```python
from build123d import *

# Parameters (mm, degrees)
BOSS_EXTRUDE1_DEPTH = 2
FILLET1_R           = 1
FILLET2_R           = 5
FILLET3_R           = 9


with BuildPart() as part:
    # Sketch1 → Boss-Extrude1 (new body)
    with BuildSketch(Plane(origin=(0, 0, 0), x_dir=(1, 0, 0), z_dir=(0, 1, 0))):
        Polygon((3, 0), (5, 0), (10, 11.071428571), (15, 0), (17, 0), (17, -5), (20, -5), (20, 0), (20, 2), (13, 17.5), (20, 33), (20, 35), (20, 40), (17, 40), (17, 35), (15, 35), (10, 23.928571429), (5, 35), (3, 35), (3, 40), (0, 40), (0, 35), (0, 33), (7, 17.5), (0, 2), (0, 0), (0, -5), (3, -5), align=None)
    extrude(amount=BOSS_EXTRUDE1_DEPTH)

    # Fillet1
    fillet1_edges = [part.edges().sort_by_distance(p)[0] for p in [
        (10, 1, -23.928571429),
        (10, 1, -11.071428571),
    ]]
    fillet(fillet1_edges, radius=FILLET1_R)

    # Fillet2
    fillet2_edges = [part.edges().sort_by_distance(p)[0] for p in [
        (7, 1, -17.5),
        (13, 1, -17.5),
    ]]
    fillet(fillet2_edges, radius=FILLET2_R)

    # Fillet3
    fillet3_edges = [part.edges().sort_by_distance(p)[0] for p in [
        (0, 1, -2),
        (0, 1, -33),
        (20, 1, -33),
        (20, 1, -2),
    ]]
    fillet(fillet3_edges, radius=FILLET3_R)


solid = part.part
```
Could you check a few things on this model? Use its own coordinates, in mm. A direction names the side the tool comes from. Give positions to 0.01 mm unless a question says otherwise; leave off trailing zeros. Loops run counter-clockwise (first coordinate to the right, second up) from the corner with the lowest first, then second, coordinate; pieces in that order, holes last. Notation, with made-up numbers: (-38.75, 53) -> (14.25, 53) arc R15 cw to (14.25, 71) -> close; hole circle Ø3 at (13.5, 34.25). An arc over 180 degrees is marked (long way). Put each result on its own line as item: value.
(1) Imagine slicing it at B-B on x = 15.75. Write out the boundary of the cut face in (y, z), plus the area to 3 significant figures.
Computed:
outline: (0, -35) -> (2, -35) -> (2, -23.59) -> (0, -23.59) -> close; (0, -11.41) -> (2, -11.41) -> (2, 0) -> (0, 0) -> close
area: 45.6 mm^2
(2) For faces 1 (the face through (16, 1, 0)), 2 (the face through (7.073, 0.986, -30.41)), 3 (the face through (0, 1, -38)), 4 (the face through (0.207, 1.014, -1.983)), 5 (the face through (16.603, 0.986, -9.522)), which set-ups out of +Z, -Z, +X, -X, +Y, -Y let a thin tool reach every point of the face, with its end or its side?
Computed:
face 1: +Z, +Y, -Y
face 2: -Z, +Y, -Y
face 3: +Z, -Z, -X, +Y, -Y
face 4: -X, +Y, -Y
face 5: +X, +Y, -Y
(3) Imagine slicing it at D-D on x = 10.5. Write out the boundary of the cut face in (y, z), plus the area to 3 significant figures.
Computed:
outline: (0, -25.49) -> (2, -25.49) -> (2, -9.51) -> (0, -9.51) -> close
area: 32.0 mm^2
(4) I'm going to push flat-ended pins straight in: pin 1 Ø0.6 at (x, y) = (16.5, 0.5) entering from -Z; pin 2 Ø0.6 at (x, y) = (4, 1) entering from +Z. Where does each tip first touch, or does it pass through?
Computed:
pin 1: z = -35
pin 2: z = 0
(5) Please list where these lines run through material, in increasing order: probe 1 along X at (y, z) = (0.7, -26); probe 2 along X at (y, z) = (0.55, -35.5); probe 3 along Z at (x, y) = (16.5, 1.35). Write a range as [from, to].
Computed:
probe 1: [3.16, 9.06], [10.94, 16.84]
probe 2: [0, 3], [17, 20]
probe 3: [-35, -25.25], [-9.75, 0]
(6) Thinking about a two-plate mould opening in Z: for faces 6 (the face through (19.804, 1.014, -1.93)), 7 (the face through (9.98, 1.01, -9.64)), 8 (the face through (0, 1, 2)), 9 (the face through (12.984, 0.986, -30.537)), which applies, pulls with the +Z half, pulls with the -Z half, needs draft (parallel to the pull), parting line crosses it, or undercut?
Computed:
face 6: undercut
face 7: pulls with the +Z half
face 8: needs draft
face 9: pulls with the -Z half
(7) Imagine slicing it at A-A on z = -37. Write out the boundary of the cut face in (x, y).
Computed:
outline: (0, 0) -> (3, 0) -> (3, 2) -> (0, 2) -> close; (17, 0) -> (20, 0) -> (20, 2) -> (17, 2) -> close
